```python
from build123d import *

# Parameters (mm, degrees)
SKETCH_1_W          = 190
SKETCH_1_H          = 42.3
EXTRUDE_1_DEPTH     = 10
SKETCH_2_W          = 42.5
SKETCH_2_H          = 77.05305565
CUT_EXTRUDE_1_DEPTH = 5
SKETCH_3_R          = 1.6
SKETCH_3_R_2        = 11.1
CUT_EXTRUDE_2_DEPTH = 6
SKETCH_4_R          = 7.55
CUT_EXTRUDE_3_DEPTH = 11
FILLET_1_R          = 5
CUT_EXTRUDE_4_REACH = 44.3
SKETCH_5_R          = 2
SKETCH_6_R          = 2
CUT_EXTRUDE_5_DEPTH = 11.0000001


with BuildPart() as part:
    # 草图1 → 凸台-拉伸1 (new body)
    with BuildSketch(Plane(origin=(0, 0, 0), x_dir=(1, 0, 0), z_dir=(0, 1, 0))):
        Rectangle(SKETCH_1_W, SKETCH_1_H)
    extrude(amount=EXTRUDE_1_DEPTH)

    # 草图2 → 切除-拉伸1 (cut)
    with BuildSketch(Plane(origin=(0, 10, 0), x_dir=(1, 0, 0), z_dir=(0, 1, 0))):
        Rectangle(SKETCH_2_W, SKETCH_2_H)
    extrude(amount=-CUT_EXTRUDE_1_DEPTH, mode=Mode.SUBTRACT)

    # 草图3 → 切除-拉伸2 (cut, through all)
    with BuildSketch(Plane(origin=(0, 5, 0), x_dir=(1, 0, 0), z_dir=(0, 1, 0))):
        with Locations((-15.5, 15.5)):
            Circle(SKETCH_3_R)
        with Locations((15.5, 15.5)):
            Circle(SKETCH_3_R)
        with Locations((15.5, -15.5)):
            Circle(SKETCH_3_R)
        with Locations((-15.5, -15.5)):
            Circle(SKETCH_3_R)
        Circle(SKETCH_3_R_2)
    extrude(amount=-CUT_EXTRUDE_2_DEPTH, mode=Mode.SUBTRACT)

    # 草图4 → 切除-拉伸3 (cut, through all)
    with BuildSketch(Plane(origin=(0, 10, 0), x_dir=(1, 0, 0), z_dir=(0, 1, 0))):
        with Locations((-85, 0)):
            Circle(SKETCH_4_R)
        with Locations((85, 0)):
            Circle(SKETCH_4_R)
    extrude(amount=-CUT_EXTRUDE_3_DEPTH, mode=Mode.SUBTRACT)

    # 圆角1
    fillet_1_edges = [part.edges().sort_by_distance(p)[0] for p in [
        (95, 5, 21.15),
        (-95, 5, 21.15),
        (-95, 5, -21.15),
        (95, 5, -21.15),
    ]]
    fillet(fillet_1_edges, radius=FILLET_1_R)

    # 草图5 → 切除-拉伸4 (cut, up to next)
    with BuildSketch(Plane.XY.offset(21.15), mode=Mode.PRIVATE) as cut_extrude_4_sk1:
        with Locations((85, 5)):
            Circle(SKETCH_5_R)
    cut_extrude_4_tool1 = extrude(cut_extrude_4_sk1.sketch, amount=-CUT_EXTRUDE_4_REACH, mode=Mode.PRIVATE) & part.part
    add(cut_extrude_4_tool1.solids().sort_by_distance((85, 5, 21.15))[0], mode=Mode.SUBTRACT)
    # 草图5 → 切除-拉伸4 (cut, up to next)
    with BuildSketch(Plane.XY.offset(21.15), mode=Mode.PRIVATE) as cut_extrude_4_sk2:
        with Locations((-85, 5)):
            Circle(SKETCH_5_R)
    cut_extrude_4_tool2 = extrude(cut_extrude_4_sk2.sketch, amount=-CUT_EXTRUDE_4_REACH, mode=Mode.PRIVATE) & part.part
    add(cut_extrude_4_tool2.solids().sort_by_distance((-85, 5, 21.15))[0], mode=Mode.SUBTRACT)

    # 草图6 → 切除-拉伸5 (cut, through all)
    with BuildSketch(Plane(origin=(0, 10, 0), x_dir=(1, 0, 0), z_dir=(0, 1, 0))):
        with Locations((-75, -16.15)):
            Circle(SKETCH_6_R)
    extrude(amount=-CUT_EXTRUDE_5_DEPTH, mode=Mode.SUBTRACT)


solid = part.part
```
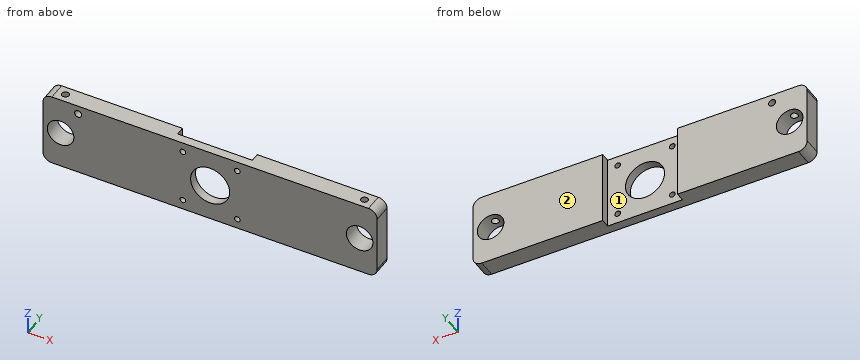
Check sheet for the modelled part. Datum: model origin and axes. Units: mm. Face numbers are marked on the shaded views. Coordinates: 2 decimals unless noted, no trailing zeros. Loops run counter-clockwise (first coordinate to the right, second up) from the corner with the lowest first, then second, coordinate; pieces in that order, holes last. Notation, with made-up numbers: M 6.25,-31 L 58.25,-31 A23 ccw 58.25,4 Z; hole C 21,-29.5 d2. An arc over 180 degrees is marked long. Answer as a JSON object with one key per item and string values.
1. Release check for a two-part mould opening along X. For the marked faces 1 and 2 record: pulls with the +X half, pulls with the -X half, needs draft (parallel to the pull), parting line crosses it, or undercut.
Outcome:
{"face 1": "undercut", "face 2": "needs draft"}
2. Sectioned sample at C-C on z = 0. Record the cut outline in (x, y), and give its area (3 significant figures).
Outcome:
{"outline": "M -95,0 L -92.55,0 L -92.55,10 L -95,10 Z; M -77.45,0 L -11.1,0 L -11.1,5 L -21.25,5 L -21.25,10 L -77.45,10 Z; M 11.1,0 L 77.45,0 L 77.45,10 L 21.25,10 L 21.25,5 L 11.1,5 Z; M 92.55,0 L 95,0 L 95,10 L 92.55,10 Z", "area": "1,270 mm²"}
3. Sectioned sample at B-B on x = -75. Record the cut outline in (y, z).
Outcome:
{"outline": "M 0,-21.15 L 10,-21.15 L 10,14.15 L 0,14.15 Z; M 0,18.15 L 10,18.15 L 10,21.15 L 0,21.15 Z"}
4. Scan lines: L1, parallel to X at y = 9, z = -0.5; L2, parallel to X at y = 2.5, z = 0; L3, parallel to X at y = 1.8, z = -15.5. Record each from-to range of solid material in increasing order. Write a range as from..to.
Outcome:
{"L1": "-95..-92.53, -77.47..-21.25, 21.25..77.47, 92.53..95", "L2": "-95..-92.55, -77.45..-11.1, 11.1..77.45, 92.55..95", "L3": "-95..-17.1, -13.9..13.9, 17.1..95"}
5. Depth check by flat-ended pin: P1, Ø5, axis at x = 15.5, z = 15.5, coming from the +Y side; P2, Ø6, axis at x = 55, z = -4, coming from the -Y side; P3, Ø2.5, axis at x = -15.5, z = -15.5, coming from the +Y side; P4, Ø2.5, axis at x = -85, y = 5, coming from the +Z side. Enter the tip coordinate at first touch or a pass-through.
Outcome:
{"P1": "y = 5", "P2": "y = 0", "P3": "through", "P4": "z = -7.45"}
6. Sectioned sample at D-D on x = 15.5. Record the cut outline in (y, z), and give its area (4 significant figures).
Outcome:
{"outline": "M 0,-21.15 L 5,-21.15 L 5,-17.1 L 0,-17.1 Z; M 0,-13.9 L 5,-13.9 L 5,13.9 L 0,13.9 Z; M 0,17.1 L 5,17.1 L 5,21.15 L 0,21.15 Z", "area": "179.5 mm²"}
7. Sectioned sample at A-A on x = 85. Record the cut outline in (y, z).
Outcome:
{"outline": "M 0,-21.15 L 10,-21.15 L 10,-7.55 L 0,-7.55 Z; M 0,7.55 L 3,7.55 L 3,21.15 L 0,21.15 Z; M 7,7.55 L 10,7.55 L 10,21.15 L 7,21.15 Z"}
